Design review of the part shown in the three views and the two pictorial views. Dimensions are in mm from the part's minimum x, y and z. Give positions to 0.01 mm unless a question says otherwise; leave off trailing zeros. Order: outer loops, then holes, each group sorted by start corner. A loop starts at its lowest first (then second) coordinate and runs counter-clockwise, first axis right, second up. Notation, with made-up numbers: (46, -39.5) - (101, -39.5) arc R16 cw to (101, -10.5) - close; hole circle Ø8 at (50.25, -15). An arc over 180 degrees is marked (long way). Put each result on its own line as item: value.
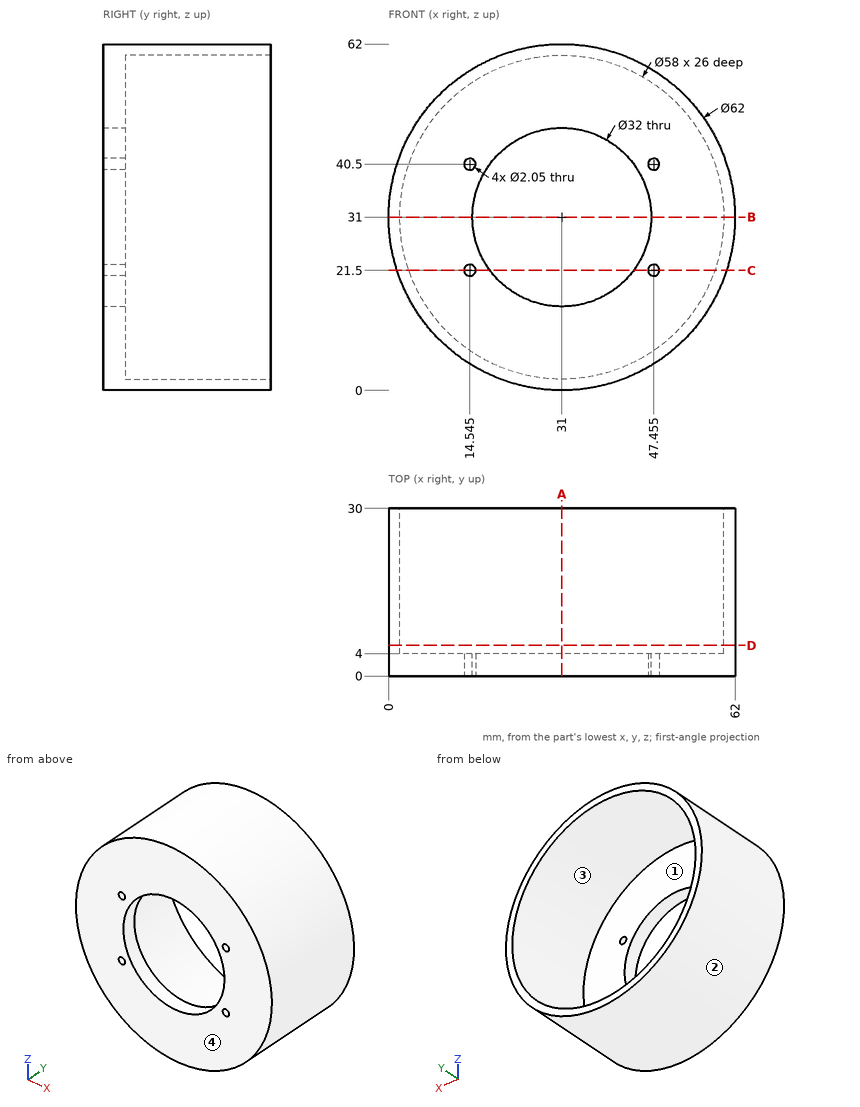
(1) Take a section at D-D, the plane y = 5.5. Write out the cut boundary in (x, z).
The answers:
outline: circle Ø62 at (31, 31); hole circle Ø58 at (31, 31)
(2) Take a section at A-A, the plane x = 31. Write out the cut boundary in (y, z).
The answers:
outline: (0, 0) - (30, 0) - (30, 2) - (4, 2) - (4, 15) - (0, 15) - close; (0, 47) - (4, 47) - (4, 60) - (30, 60) - (30, 62) - (0, 62) - close
(3) Clearance check with flat-ended pins moving along their axes: pin 1 Ø12 at (y, z) = (26, 10) entering from +X; pin 2 Ø5 at (x, y) = (42.5, 11) entering from +Z; pin 3 Ø2.5 at (x, z) = (47.455, 21.5) entering from +Y. State where each tip first meets the part, or that it passes through.
The answers:
pin 1: x = 58.13
pin 2: z = 60.66
pin 3: y = 4
(4) Take a section at C-C, the plane z = 21.5. Write out the cut boundary in (x, y), then the cut area to 3 significant figures.
The answers:
outline: (1.49, 0) - (13.52, 0) - (13.52, 4) - (3.6, 4) - (3.6, 30) - (1.49, 30) - close; (15.57, 0) - (18.13, 0) - (18.13, 4) - (15.57, 4) - close; (43.87, 0) - (46.43, 0) - (46.43, 4) - (43.87, 4) - close; (48.48, 0) - (60.51, 0) - (60.51, 30) - (58.4, 30) - (58.4, 4) - (48.48, 4) - close
area: 226 mm^2
(5) The part is to be moulded in two halves that separate along X. For the marked faces 1, 2, 3 and 4, say which applies: pulls with the +X half, pulls with the -X half, needs draft (parallel to the pull), parting line crosses it, or undercut.
The answers:
face 1: undercut
face 2: parting line crosses it
face 3: undercut
face 4: needs draft
(6) Wall thickness on L1, parallel to X at y = 2.3, z = 31; L2, parallel to X at y = 2.6, z = 21.5; L3, parallel to Y at x = 39.5, z = 9: over which ranges is each line inside the solid? List them lowest first.
The answers:
L1: 0 to 15, 47 to 62
L2: 1.49 to 13.52, 15.57 to 18.13, 43.87 to 46.43, 48.48 to 60.51
L3: 0 to 4
(7) Take a section at B-B, the plane z = 31. Write out the cut boundary in (x, y), then the cut area to 3 significant figures.
The answers:
outline: (0, 0) - (15, 0) - (15, 4) - (2, 4) - (2, 30) - (0, 30) - close; (47, 0) - (62, 0) - (62, 30) - (60, 30) - (60, 4) - (47, 4) - close
area: 224 mm^2
